Could you check a few things on this model? Use its own coordinates, in mm. Coordinates: 2 decimals unless noted, no trailing zeros. Loops run counter-clockwise (first coordinate to the right, second up) from the corner with the lowest first, then second, coordinate; pieces in that order, holes last.
1) Imagine slicing it at D-D on x = -21. Please give me the cut outline in (y, z).
2) Thinking about a two-plate mould opening in Y: for faces 1 (the face through (-6, 3, -1)), 2 (the face through (-6, -3, -1)), 3 (the face through (-41.667, 0.601, -1.059)), 4 (the face through (-46.574, 0.066, -1.113)), which applies, released by +Y, released by -Y, zero draft, split by the parting line, or undercut?
3) If I drill on line 1 along X through (y, z) = (-0.1, -41.5); line 2 along X through (y, z) = (1, -23); line 3 along Y through (x, z) = (29.5, -53), over which ranges is the centre line in solid material (lowest first)?
4) Will these pins go through, and if not, where does the flat tip stop? P1, Ø1.5, axis at y = -2, z = 29, coming from the -X side; P2, Ø1.5, axis at x = 13, y = -2, coming from the +Z side; P3, Ø2.5, axis at x = 30.43, y = 0, coming from the -Z side.
5) Imagine slicing it at B-B on y = 0. Please give me the cut outline in (x, z).
6) Imagine slicing it at A-A on z = -34. Please give me the cut outline in (x, y), plus the area to 3 significant figures.
7) Imagine slicing it at C-C on z = 47. Please give me the cut outline in (x, y).
```python
from build123d import *

# Parameters (mm, degrees)
BOSS_EXTRUDE1_DEPTH = 3
BOSS_EXTRUDE2_REACH = 76.759
SKETCH2_R           = 3
BOSS_EXTRUDE3_REACH = 79.18
SKETCH2_3_R         = 3
SKETCH2_3_R_2       = 2
SKETCH2_4_R         = 2
CUT_EXTRUDE1_DEPTH  = 103


with BuildPart() as part:
    # Sketch1 → Boss-Extrude1 (new, symmetric)
    with BuildSketch(Plane(origin=(0, 0, 0), x_dir=(1, 0, 0), z_dir=(0, 1, 0))):
        Polygon((-43.574876661, -41), (-43.574876661, 0), (30.425123339, 0), (30.425123339, -60.672481425), align=None)
        Polygon((-43.574876661, 44.4209239), (30.425123339, 60.672481425), (30.425123339, 0), (-43.574876661, 0), align=None)
    extrude(amount=BOSS_EXTRUDE1_DEPTH, both=True)

    # Boss-Extrude2: up to this plane
    boss_extrude2_end = Plane(origin=(-13.056453191, 3, 49.113150255), z_dir=(0.2569206163076567, 0, -0.9664325102748219))
    # Sketch2 → Boss-Extrude2 (add, up to the surface)
    with BuildSketch(Plane.XY, mode=Mode.PRIVATE) as boss_extrude2_sk1:
        with Locations((30.425123339, 0)):
            Circle(SKETCH2_R)
    boss_extrude2_tool1 = split(extrude(boss_extrude2_sk1.sketch, amount=BOSS_EXTRUDE2_REACH, mode=Mode.PRIVATE), bisect_by=boss_extrude2_end, keep=Keep.BOTH, mode=Mode.PRIVATE)
    add(boss_extrude2_tool1.solids().sort_by_distance((30.425123, 0, 0))[0])
    # Sketch2 → Boss-Extrude2 (add, up to the surface)
    with BuildSketch(Plane.XY, mode=Mode.PRIVATE) as boss_extrude2_sk2:
        with Locations((-43.574876661, 0)):
            Circle(SKETCH2_R)
    boss_extrude2_tool2 = split(extrude(boss_extrude2_sk2.sketch, amount=BOSS_EXTRUDE2_REACH, mode=Mode.PRIVATE), bisect_by=boss_extrude2_end, keep=Keep.BOTH, mode=Mode.PRIVATE)
    add(boss_extrude2_tool2.solids().sort_by_distance((-43.574877, 0, 0))[0])

    # Boss-Extrude3: up to this plane
    boss_extrude3_end = Plane(origin=(-11.311619848, 3, -51.506439766), z_dir=(-0.21450368815955828, 0, -0.9767231786775346))
    # Sketch2_3 → Boss-Extrude3 (add, up to the surface)
    with BuildSketch(Plane.XY, mode=Mode.PRIVATE) as boss_extrude3_sk1:
        with Locations((30.425123339, 0)):
            Circle(SKETCH2_3_R)
        with Locations((30.425123339, 0)):
            Circle(SKETCH2_3_R_2, mode=Mode.SUBTRACT)
    boss_extrude3_tool1 = split(extrude(boss_extrude3_sk1.sketch, amount=-BOSS_EXTRUDE3_REACH, mode=Mode.PRIVATE), bisect_by=boss_extrude3_end, keep=Keep.BOTH, mode=Mode.PRIVATE)
    add(boss_extrude3_tool1.solids().sort_by_distance((27.509976, 0, 0))[0])
    # Sketch2_3 → Boss-Extrude3 (add, up to the surface)
    with BuildSketch(Plane.XY, mode=Mode.PRIVATE) as boss_extrude3_sk2:
        with Locations((-43.574876661, 0)):
            Circle(SKETCH2_3_R)
        with Locations((-43.574876661, 0)):
            Circle(SKETCH2_3_R_2, mode=Mode.SUBTRACT)
    boss_extrude3_tool2 = split(extrude(boss_extrude3_sk2.sketch, amount=-BOSS_EXTRUDE3_REACH, mode=Mode.PRIVATE), bisect_by=boss_extrude3_end, keep=Keep.BOTH, mode=Mode.PRIVATE)
    add(boss_extrude3_tool2.solids().sort_by_distance((-46.490024, 0, 0))[0])

    # Sketch2_4 → Cut-Extrude1 (cut, symmetric)
    with BuildSketch(Plane.XY):
        with Locations((30.425123339, 0)):
            Circle(SKETCH2_4_R)
        with Locations((-43.574876661, 0)):
            Circle(SKETCH2_4_R)
    extrude(amount=CUT_EXTRUDE1_DEPTH, both=True, mode=Mode.SUBTRACT)


solid = part.part
```
Filled in:
1. outline: (-3, -49.38) - (3, -49.38) - (3, 47) - (-3, 47) - close
2. face 1: released by +Y
2. face 2: released by -Y
2. face 3: undercut
2. face 4: split by the parting line
3. line 1: x = -46.57 to -45.57, -41.58 to 28.43, 32.42 to 33.42
3. line 2: x = -46.4 to -45.31, -41.84 to 28.69, 32.16 to 33.25
3. line 3: y = -3 to -1.77, 1.77 to 3
4. P1: stops at x = -46.3
4. P2: stops at z = 56.24
4. P3: passes through
5. outline: (-46.57, -43.76) - (-45.57, -43.98) - (-45.57, 40.47) - (-46.57, 40.2) - close; (-41.57, -44.86) - (28.43, -60.23) - (28.43, 60.14) - (-41.57, 41.53) - close; (32.43, -61.11) - (33.43, -61.33) - (33.43, 61.47) - (32.43, 61.2) - close
6. outline: (-43.57, -3) - (30.43, -3) arc R3 ccw to (30.43, 3) - (-43.57, 3) arc R3 ccw to start; hole circle Ø4 at (-43.57, 0); hole circle Ø4 at (30.43, 0)
6. area: 447 mm2
7. outline: (-21.01, -3) - (30.43, -3) arc R3 ccw to (30.43, 3) - (-21.01, 3) - close; hole circle Ø4 at (30.43, 0)
